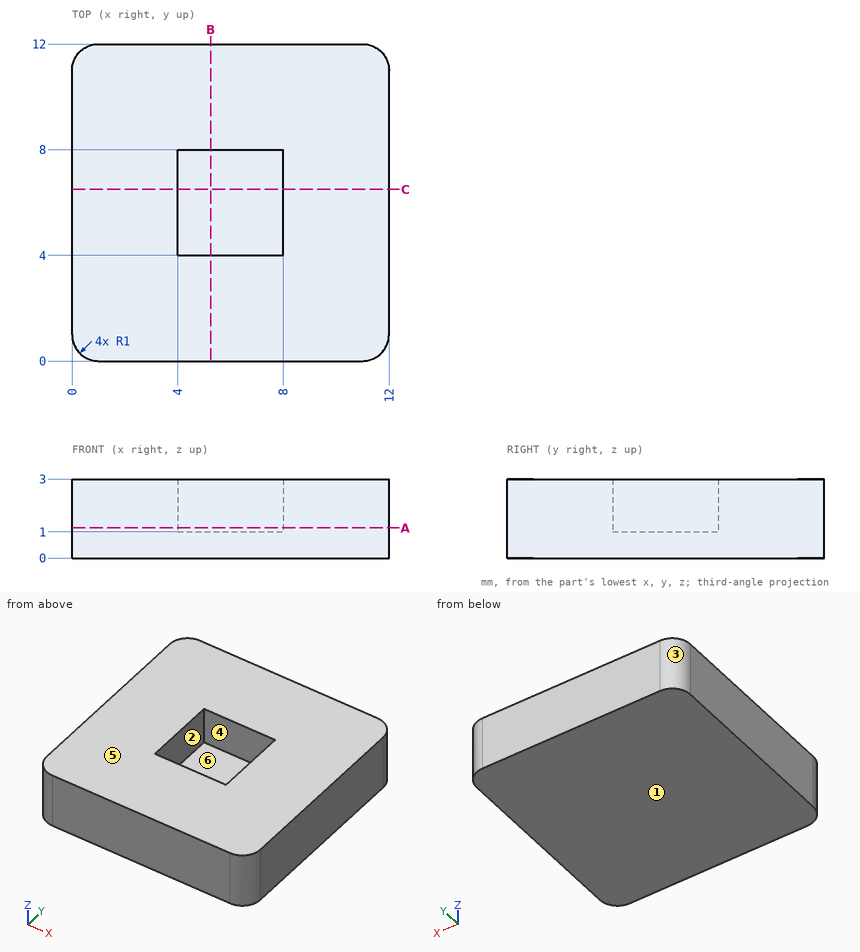
Here's the drawing with two shaded views (mm, measured from the low corner). I have some questions. A direction names the side the tool comes from. Give positions to 0.01 mm unless a question says otherwise; leave off trailing zeros. Order: outer loops, then holes, each group sorted by start corner. A loop starts at its lowest first (then second) coordinate and runs counter-clockwise, first axis right, second up. Notation, with made-up numbers: (-10.75, -29) - (6.25, -29) arc R19 cw to (6.25, -1) - close; hole circle Ø5 at (-28, -1.5). An arc over 180 degrees is marked (long way). Use a Markdown table: item, result. Add a question column.
Q1. If we section it at B-B on x = 5.25: Write out the boundary of the cut face in (y, z).
Q2. If we section it at A-A on z = 1.15: Write out the boundary of the cut face in (x, y), plus the area to 3 significant figures.
Q3. If we mould it in two halves opening along Y, with no side actions, what happens to the marked faces 1, 2, 3 and 4? For each: released by +Y, released by -Y, zero draft, split by the parting line, or undercut.
Q4. On a 3-axis mill with a long thin cutter (end or side, diameter ignored), from which of +Z, -Z, +X, -X, +Y, -Y can I reach the whole of each face in a straight line? I mean the marked faces 5 and 6. Say none if no direction works.
Q5. Please list where these lines run through material, in increasing order: line 1 along Y through (x, z) = (6, 1.45); line 2 along Z through (x, y) = (6.25, 6).
Answers follow:
| question | item | result |
|---|---|---|
| 1 | outline | (0, 0) - (12, 0) - (12, 3) - (8, 3) - (8, 1) - (4, 1) - (4, 3) - (0, 3) - close |
| 2 | outline | (0, 1) arc R1 ccw to (1, 0) - (11, 0) arc R1 ccw to (12, 1) - (12, 11) arc R1 ccw to (11, 12) - (1, 12) arc R1 ccw to (0, 11) - close; hole (4, 4) - (8, 4) - (8, 8) - (4, 8) - close |
| 2 | area | 127 mm^2 |
| 3 | face 1 | zero draft |
| 3 | face 2 | undercut |
| 3 | face 3 | released by +Y |
| 3 | face 4 | undercut |
| 4 | face 5 | +Z, +X, -X, +Y, -Y |
| 4 | face 6 | +Z |
| 5 | line 1 | y = 0 to 4, 8 to 12 |
| 5 | line 2 | z = 0 to 1 |
